Geometry: see drawing. Coordinates: mm, zero at the bounding-box minimum. A direction names the side the tool comes from. Round coordinates to 2 decimals unless told otherwise and drop trailing zeros. Loops run counter-clockwise (first coordinate to the right, second up) from the corner with the lowest first, then second, coordinate; pieces in that order, holes last. Notation, with made-up numbers: (40.25, 65.5) - (93.25, 65.5) arc R12 cw to (93.25, 80.5) - close; hole circle Ø5 at (49, 1). An arc over 180 degrees is marked (long way). Use CSV: the item, a comma, the result in double quotes.
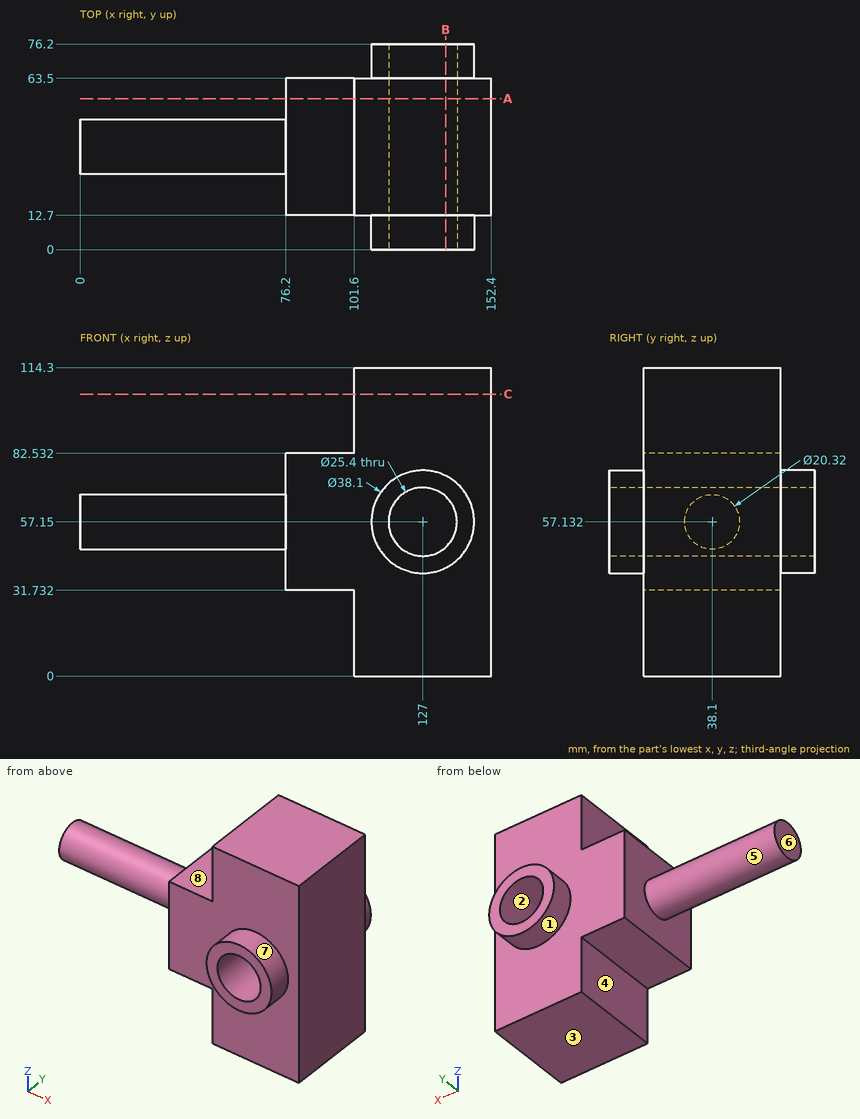
Item 1: Mould query, pull axis X, two halves, no side actions, for the marked faces 1, 2 and 3. Classes: released by +X, released by -X, zero draft, split by the parting line, or undercut.
Final values:
face 1,"split by the parting line"
face 2,"undercut"
face 3,"zero draft"
Item 2: Section C-C on z = 104.5. Return the cut outline in (x, y).
Final values:
outline,"(101.6, 12.7) - (152.4, 12.7) - (152.4, 63.5) - (101.6, 63.5) - close"
Item 3: Pin query (flat end, axial travel): P1, Ø20.5, axis at x = 84, y = 50.5, coming from the +Z side; P2, Ø7.5, axis at x = 89.5, y = 35.5, coming from the -Z side; P3, Ø9.5, axis at y = 37.5, z = 102, coming from the -X side; P4, Ø20.5, axis at x = 127, z = 57.15, coming from the +Y side. Return the tip coordinate at first contact, or that it passes through.
Final values:
P1,"stops at z = 82.53"
P2,"stops at z = 31.73"
P3,"stops at x = 101.6"
P4,"passes through"
Item 4: Reachability of the marked faces 4, 5, 6, 7 and 8 from +Z, -Z, +X, -X, +Y, -Y: full face, straight path, thin tool, end or side. Return the list, or none.
Final values:
face 4,"-Z, -X, +Y, -Y"
face 5,"-X"
face 6,"+Z, -Z, -X, +Y, -Y"
face 7,"-Y"
face 8,"+Z, -X, +Y, -Y"
Item 5: Section B-B on x = 135.5. Return the cut outline in (y, z).
Final values:
outline,"(0, 40.1) - (12.7, 40.1) - (12.7, 0) - (63.5, 0) - (63.5, 40.1) - (76.2, 40.1) - (76.2, 47.71) - (0, 47.71) - close; (0, 66.59) - (76.2, 66.59) - (76.2, 74.2) - (63.5, 74.2) - (63.5, 114.3) - (12.7, 114.3) - (12.7, 74.2) - (0, 74.2) - close"
Item 6: Section A-A on y = 56. Return the cut outline in (x, z), plus the area to 3 significant figures.
Final values:
outline,"(76.2, 31.73) - (101.6, 31.73) - (101.6, 0) - (152.4, 0) - (152.4, 114.3) - (101.6, 114.3) - (101.6, 82.53) - (76.2, 82.53) - close; hole circle Ø25.4 at (127, 57.15)"
area,"6,590 mm²"
Item 7: Material intervals for line 1 (X direction, y = 17, z = 57); line 2 (Z direction, x = 127, y = 49); line 3 (X direction, y = 53, z = 29.5), sorted ascending.
Final values:
line 1,"x = 76.2 to 114.3, 139.7 to 152.4"
line 2,"z = 0 to 44.45, 69.85 to 114.3"
line 3,"x = 101.6 to 152.4"
